Autodesk Fusion 360 part; units mm, degrees
sketch "Sketch1" plane through (0, 0, 0) normal (0, 0, 1) x (1, 0, 0)
  line L0 (-20, 20) -> (60, 20)
  line L1 (60, 20) -> (60, -30)
  line L2 (60, -30) -> (-20, -30)
  line L3 (-20, -30) -> (-20, 20)
  dimension "d1" = 80
  dimension "d2" = 50
extrude "Extrude1" add sketch "Sketch1" along normal blind 80
cylinder "CylinderPrimitive1" cut diameter 28 height -100 placed x (0, 0, -1) y (0, 1, 0) z (1, 0, 0) at (60, -5, 25)
cylinder "CylinderPrimitive2" cut diameter 28 height -95 placed x (0, 0, -1) y (0, 1, 0) z (1, 0, 0) at (60, -5, 60)
box "BoxPrimitive1" cut length 73.4567 width 43.5237 height -75 placed x (0, 0, -1) y (0, -1, 0) z (-1, 0, 0) at (-20, 16.7884, 76.3145)
cylinder "CylinderPrimitive3" cut diameter 2.84 height -65 placed x (1, 0, 0) y (0, 0, 1) z (0, -1, 0) at (25, -30, 45)
The model under review builds one solid part; all positions refer to its coordinate system, in mm. A direction names the side the tool comes from. Round coordinates to 2 decimals unless told otherwise and drop trailing zeros. Loops run counter-clockwise (first coordinate to the right, second up) from the corner with the lowest first, then second, coordinate; pieces in that order, holes last. Notation, with made-up numbers: (60.25, -35.75) - (113.25, -35.75) arc R19 ccw to (113.25, -26.75) - close; hole circle Ø9 at (-28, -33). An arc over 180 degrees is marked (long way). Use a Markdown table: item, result. Add a question column.
Q1. Add section D-D (z = 45). State the section outline as (x, y) points, plus the area to 3 significant figures.
Q2. Add section A-A (x = 25). State the section outline as (y, z) points.
Q3. Add section B-B (z = 60). State the section outline as (x, y) points.
Q4. Machinability: for faces 5 (the face through (21, -30, 39)), 6 (the face through (18, -5, 2.858)), which of the approach directions +Z, -Z, +X, -X, +Y, -Y give a long, thin tool a straight path to every point of the face, cutting with its end or side? Answer none if there is none.
Q5. Insertion check: pin 1 Ø8 at (y, z) = (-17.5, 62.5) entering from -X; pin 2 Ø25 at (y, z) = (-5, 25) entering from -X. Each pin has a flat end and moves straight along its axis. Give the tip position at first contact, or say it passes through.
Q6. For probe 1 along Y at (x, z) = (58, 60); probe 2 along Y at (x, z) = (15, 60); probe 3 along Z at (x, y) = (18, 15.5), list the stretches that pass through material, from the lowest coordinate up.
Q7. The part is to be moulded in two halves that separate along Z. For faces 1 (the face through (19, -5, 0)), 2 (the face through (57.54, -18.67, 28.03)), 3 (the face through (18, -26.735, 39)), 4 (the face through (60, -4.7, 39.4)), say which applies: pulls with the +Z half, pulls with the -Z half, needs draft (parallel to the pull), parting line crosses it, or undercut.
Q8. Add section C-C (y = -5). State the section outline as (x, z) points, plus the area to 3 significant figures.
Worked answers:
| question | item | result |
|---|---|---|
| 1 | outline | (-20, -30) - (23.58, -30) - (23.58, -26.74) - (-20, -26.74) - close; (-20, 16.79) - (23.58, 16.79) - (23.58, 20) - (-20, 20) - close; (26.42, -30) - (60, -30) - (60, 20) - (26.42, 20) - (26.42, 16.79) - (55, 16.79) - (55, -26.74) - (26.42, -26.74) - close |
| 1 | area | 717 mm² |
| 2 | outline | (-30, 0) - (20, 0) - (20, 43.58) - (16.79, 43.58) - (16.79, 2.86) - (-26.74, 2.86) - (-26.74, 43.58) - (-30, 43.58) - close; (-30, 46.42) - (-26.74, 46.42) - (-26.74, 76.31) - (16.79, 76.31) - (16.79, 46.42) - (20, 46.42) - (20, 80) - (-30, 80) - close |
| 3 | outline | (-20, -30) - (60, -30) - (60, -19) - (55, -19) - (55, -26.74) - (-20, -26.74) - close; (-20, 16.79) - (55, 16.79) - (55, 9) - (60, 9) - (60, 20) - (-20, 20) - close |
| 4 | face 5 | +Z, -Z, +X, -X, -Y |
| 4 | face 6 | -X |
| 5 | pin 1 | x = 55 |
| 5 | pin 2 | through |
| 6 | probe 1 | -30 to -19, 9 to 20 |
| 6 | probe 2 | -30 to -26.74, 16.79 to 20 |
| 6 | probe 3 | 0 to 2.86, 76.31 to 80 |
| 7 | face 1 | pulls with the -Z half |
| 7 | face 2 | undercut |
| 7 | face 3 | undercut |
| 7 | face 4 | needs draft |
| 8 | outline | (-20, 0) - (60, 0) - (60, 11) - (55, 11) - (55, 2.86) - (-20, 2.86) - close; (-20, 76.31) - (55, 76.31) - (55, 74) - (60, 74) - (60, 80) - (-20, 80) - close; (55, 39) - (60, 39) - (60, 46) - (55, 46) - close |
| 8 | area | 611 mm² |
